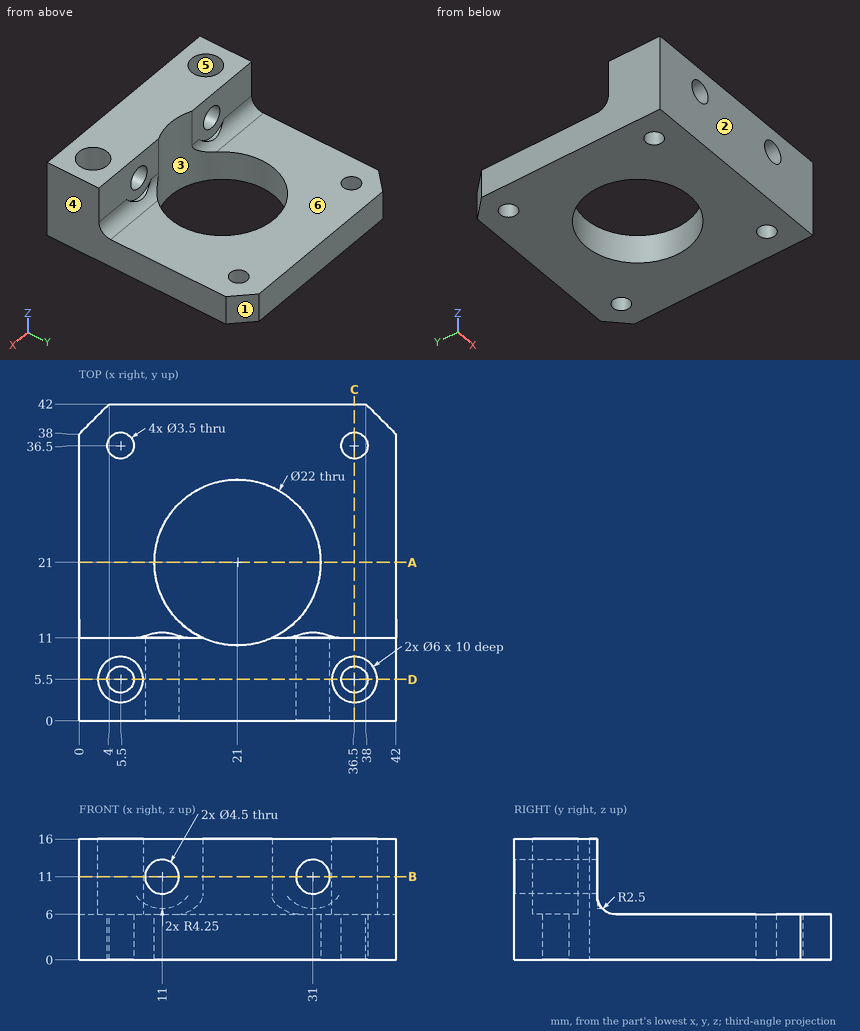
Geometry: see drawing. Coordinates: mm, zero at the bounding-box minimum. A direction names the side the tool comes from. Round coordinates to 2 decimals unless told otherwise and drop trailing zeros. Order: outer loops, then holes, each group sorted by start corner. A loop starts at its lowest first (then second) coordinate and runs counter-clockwise, first axis right, second up. Notation, with made-up numbers: (63.25, 40.25) -> (95.25, 40.25) arc R18 cw to (95.25, 74.25) -> close; hole circle Ø9 at (28, 77.5). An arc over 180 degrees is marked (long way). Answer as CSV lines item,"result".
Item 1: Line query: L1, parallel to Y at x = 5.5, z = 1.2; L2, parallel to Y at x = 21, z = 2.5; L3, parallel to X at y = 4.5, z = 9.5. Output: solid intervals per line, ascending.
A:
L1,"0 to 3.75, 7.25 to 34.75, 38.25 to 42"
L2,"0 to 10, 32 to 42"
L3,"0 to 2.67, 8.33 to 9.32, 12.68 to 29.32, 32.68 to 33.67, 39.33 to 42"
Item 2: Pull-direction query (Y, two-part tool) for the marked faces 1, 2 and 3; classes: pulls with the +Y half, pulls with the -Y half, needs draft (parallel to the pull), parting line crosses it, or undercut.
A:
face 1,"pulls with the +Y half"
face 2,"pulls with the -Y half"
face 3,"undercut"
Item 3: Section B-B, the plane z = 11. Return loops of the section in (x, y), plus the area to 3 significant figures.
A:
outline,"(0, 0) -> (8.75, 0) -> (8.75, 11) -> (0, 11) -> close; (13.25, 0) -> (28.75, 0) -> (28.75, 11) -> (25.58, 11) arc R11 cw to (16.42, 11) -> (13.25, 11) -> close; (33.25, 0) -> (42, 0) -> (42, 11) -> (33.25, 11) -> close; hole circle Ø6 at (5.5, 5.5); hole circle Ø6 at (36.5, 5.5)"
area,"300 mm²"
Item 4: Pin query (flat end, axial travel): pin 1 Ø5.5 at (x, y) = (36.5, 36.5) entering from +Z; pin 2 Ø4.5 at (x, z) = (35, 10.5) entering from +Y. Return the tip coordinate at first contact, or that it passes through.
A:
pin 1,"z = 6"
pin 2,"y = 11.01"
Item 5: Section A-A, the plane y = 21. Return loops of the section in (x, z), plus the area to 3 significant figures.
A:
outline,"(0, 0) -> (10, 0) -> (10, 6) -> (0, 6) -> close; (32, 0) -> (42, 0) -> (42, 6) -> (32, 6) -> close"
area,"120 mm²"
Item 6: Section D-D, the plane y = 5.5. Return loops of the section in (x, z).
A:
outline,"(0, 0) -> (3.75, 0) -> (3.75, 6) -> (2.5, 6) -> (2.5, 16) -> (0, 16) -> close; (7.25, 0) -> (34.75, 0) -> (34.75, 6) -> (33.5, 6) -> (33.5, 16) -> (8.5, 16) -> (8.5, 6) -> (7.25, 6) -> close; (38.25, 0) -> (42, 0) -> (42, 16) -> (39.5, 16) -> (39.5, 6) -> (38.25, 6) -> close; hole circle Ø4.5 at (11, 11); hole circle Ø4.5 at (31, 11)"
Item 7: Section C-C, the plane x = 36.5. Return loops of the section in (y, z), plus the area to 3 significant figures.
A:
outline,"(0, 0) -> (3.75, 0) -> (3.75, 6) -> (2.5, 6) -> (2.5, 16) -> (0, 16) -> close; (7.25, 0) -> (34.75, 0) -> (34.75, 6) -> (13.5, 6) arc R2.5 cw to (11, 8.5) -> (11, 16) -> (8.5, 16) -> (8.5, 6) -> (7.25, 6) -> close; (38.25, 0) -> (42, 0) -> (42, 6) -> (38.25, 6) -> close"
area,"261 mm²"
Item 8: Reachability of the marked faces 4, 5 and 6 from +Z, -Z, +X, -X, +Y, -Y: full face, straight path, thin tool, end or side. Return the list, or none.
A:
face 4,"+Z, -Z, +X, +Y, -Y"
face 5,"+Z"
face 6,"+Z, +X, -X, +Y"
